```python
from build123d import *

# Parameters (mm, degrees)
SKETCH_W            = 24
SKETCH_H            = 42
PAD_DEPTH           = 22
SKETCH001_W         = 20
SKETCH001_H         = 38
POCKET_DEPTH        = 20
SKETCH002_W         = 20
SKETCH002_H         = 6
POCKET001_DEPTH     = 5
POCKET001_FACE4_W   = 42
POCKET001_FACE4_H   = 24
POCKET001_FACE4_W_2 = 6
POCKET001_FACE4_H_2 = 20
PAD001_DEPTH        = 20
CHAMFER_SIZE        = 19.9
PAD002_DEPTH        = 40
FILLET_R            = 3
FILLET001_R         = 0.9
SKETCH004_W         = 40
SKETCH004_H         = 37
PAD003_DEPTH        = 20
FILLET002_R         = 1
CHAMFER001_SIZE     = 7.9
CHAMFER002_SIZE     = 11


with BuildPart() as part:
    # Sketch → Pad (new body)
    with BuildSketch(Plane.XY):
        with Locations((0, 24)):
            Rectangle(SKETCH_W, SKETCH_H)
    extrude(amount=PAD_DEPTH)

    # Sketch001 (on Face6 of Pad) → Pocket (cut)
    with BuildSketch(Plane.XY.offset(22)):
        with Locations((0, 24)):
            Rectangle(SKETCH001_W, SKETCH001_H)
    extrude(amount=-POCKET_DEPTH, mode=Mode.SUBTRACT)

    # Sketch002 (on Face11 of Pocket) → Pocket001 (cut)
    with BuildSketch(Plane.XY.offset(2)):
        with Locations((0, 14)):
            Rectangle(SKETCH002_W, SKETCH002_H)
    extrude(amount=-POCKET001_DEPTH, mode=Mode.SUBTRACT)

    # Pocket001 Face4 → Pad001 (add)
    with BuildSketch(Plane(origin=(0, 25.351351, 0), x_dir=(0, -1, 0), z_dir=(0, 0, -1))):
        with Locations((1.351351, 0)):
            Rectangle(POCKET001_FACE4_W, POCKET001_FACE4_H)
        with Locations((11.351351, 0)):
            Rectangle(POCKET001_FACE4_W_2, POCKET001_FACE4_H_2, mode=Mode.SUBTRACT)
    extrude(amount=PAD001_DEPTH)

    # Chamfer
    chamfer_edges = [part.edges().sort_by_distance(p)[0] for p in [
        (0, 45, -20),
    ]]
    chamfer(chamfer_edges, length=CHAMFER_SIZE)

    # Sketch003 (on Face8 of Chamfer) → Pad002 (join)
    with BuildSketch(Plane.XZ.offset(-3)):
        with BuildLine():
            Line((12, -20), (-12, -20))
            add(Edge.make_bspline(
                [(-12, -20), (0, 0), (12, -20)],
                knots=[0, 0, 0, 1, 1, 1], degree=2))
        make_face()
    extrude(amount=PAD002_DEPTH)

    # Fillet
    fillet_edges = [part.edges().sort_by_distance(p)[0] for p in [
        (-0.002974, -37, -10.000001),
    ]]
    fillet(fillet_edges, radius=FILLET_R)

    # Fillet001
    fillet001_edges = [part.edges().sort_by_distance(p)[0] for p in [
        (0, 45, 22),
        (-12, 24, 22),
        (12, 24, 22),
        (0, 3, 22),
        (0, 43, 22),
        (10, 24, 22),
        (0, 5, 22),
        (-10, 24, 22),
    ]]
    fillet(fillet001_edges, radius=FILLET001_R)

    # Sketch004 (on Face21 of Fillet001) → Pad003 (join)
    with BuildSketch(Plane(origin=(0, 0, -20), x_dir=(1, 0, 0), z_dir=(0, 0, -1))):
        with Locations((0, 18.5)):
            Rectangle(SKETCH004_W, SKETCH004_H)
    extrude(amount=PAD003_DEPTH)

    # Fillet002
    fillet002_edges = [part.edges().sort_by_distance(p)[0] for p in [
        (0, -37, -40),
        (20, -18.5, -40),
        (0, 0, -40),
        (-20, -18.5, -40),
    ]]
    fillet(fillet002_edges, radius=FILLET002_R)

    # Chamfer001
    chamfer001_edges = [part.edges().sort_by_distance(p)[0] for p in [
        (-20, -18.5, -20),
        (20, -18.5, -20),
    ]]
    chamfer(chamfer001_edges, length=CHAMFER001_SIZE)

    # Chamfer002
    chamfer002_edges = [part.edges().sort_by_distance(p)[0] for p in [
        (20, -18.5, -27.9),
        (-20, -18.5, -27.9),
    ]]
    chamfer(chamfer002_edges, length=CHAMFER002_SIZE)


solid = part.part
```
Part model, mm, in its own coordinate system. A direction names the side the tool comes from. Coordinates: 2 decimals unless noted, no trailing zeros. Order: outer loops, then holes, each group sorted by start corner. A loop starts at its lowest first (then second) coordinate and runs counter-clockwise, first axis right, second up. Notation, with made-up numbers: (69, 47.25) -> (110, 47.25) arc R11 cw to (110, 60.25) -> close; hole circle Ø11 at (18.25, 6.5). An arc over 180 degrees is marked (long way). Put each result on its own line as item: value. Start each with the question number.
(1) Band-saw the part on B-B (z = -2). Give the cut face in (x, y), then the cut area to 3 significant figures.
(2) Band-saw the part on A-A (y = 8). Give the cut face in (x, z), then the cut area to 3 significant figures.
(3) Mould opens along X. For faces 4 (the face through (-16.056, -18.241, -29.379)), 5 (the face through (0, 11, -9)), 6 (the face through (12, 24, 1)) say: pulls with the +X half, pulls with the -X half, needs draft (parallel to the pull), parting line crosses it, or undercut.
(4) Probe line 1 along Y through (x, z) = (2.5, 13.5); line 2 along Y through (x, z) = (8.5, -35); line 3 along Z through (x, y) = (-9.5, 17.5). List the from-to ranges inside material, lowest first. Write a range as [from, to].
(5) Band-saw the part on C-C (z = 5). Give the cut face in (x, y), then the cut area to 3 significant figures.
(6) Band-saw the part on D-D (x = -17). Give the cut face in (y, z), then the cut area to 3 significant figures.
(7) Which spindle directions (+Z, -Z, +X, -X, +Y, -Y) get a long thin tool onto all of the face, cutting with end or side? Do faces 1 (the face through (0, 0, -29)), 2 (the face through (0, -19, -40)), 3 (the face through (0, 5, 12)). Say none if no direction does.
(8) Pin check, flat tips, straight feed: pin 1 Ø15 at (x, z) = (6.5, -29.5) entering from +Y; pin 2 Ø6 at (x, y) = (-3.5, 35) entering from +Z; pin 3 Ø9.5 at (x, z) = (2.5, 7) entering from -Y; pin 4 Ø1.5 at (y, z) = (-12, -7.5) entering from +X. Stop position of each tip, or through.
Determined:
1. outline: (-12, 3) -> (12, 3) -> (12, 43.1) -> (-12, 43.1) -> close; hole (-10, 11) -> (10, 11) -> (10, 17) -> (-10, 17) -> close
1. area: 842 mm²
2. outline: (-12, -20) -> (12, -20) -> (12, 21.1) arc R0.9 ccw to (11.1, 22) -> (10.9, 22) arc R0.9 ccw to (10, 21.1) -> (10, 2) -> (-10, 2) -> (-10, 21.1) arc R0.9 ccw to (-10.9, 22) -> (-11.1, 22) arc R0.9 ccw to (-12, 21.1) -> close
2. area: 607 mm²
3. face 4: pulls with the -X half
3. face 5: undercut
3. face 6: pulls with the +X half
4. line 1: y = [3, 5], [43, 45]
4. line 2: y = [-37, 0]
4. line 3: z = [-20, 2]
5. outline: (-12, 3) -> (12, 3) -> (12, 45) -> (-12, 45) -> close; hole (-10, 5) -> (10, 5) -> (10, 43) -> (-10, 43) -> close
5. area: 248 mm²
6. outline: (-37, -39) arc R1 ccw to (-36, -40) -> (-1, -40) arc R1 ccw to (0, -39) -> (0, -31.66) -> (-37, -31.66) -> close
6. area: 308 mm²
7. face 1: -Z, +X, -X, +Y
7. face 2: -Z, +X, -X, +Y, -Y
7. face 3: +Z
8. pin 1: stops at y = 0
8. pin 2: stops at z = 2
8. pin 3: stops at y = 3
8. pin 4: passes through
